from build123d import *

# Parameters (mm, degrees)
SKETCH1_W           = 944
SKETCH1_H           = 20
BOSS_EXTRUDE1_DEPTH = 204
CUT_EXTRUDE1_DEPTH  = 18
CUT_EXTRUDE2_DEPTH  = 2


with BuildPart() as part:
    # Sketch1 → Boss-Extrude1 (new body)
    with BuildSketch(Plane.XY):
        with Locations((393.099899989, 5.665003505)):
            Rectangle(SKETCH1_W, SKETCH1_H)
    extrude(amount=-BOSS_EXTRUDE1_DEPTH)

    # 3DSketch1 → Cut-Extrude1 (cut)
    with BuildSketch(Plane(origin=(863.099899989, 15.665003505, -202), x_dir=(-0.9781059289848355, 0, 0.2081076444648586), z_dir=(0, -1, 0))):
        Polygon((0, 0), (919.419573246, 195.621185797), (961.041102139, 0), (41.621528893, -195.621185797), align=None)
    extrude(amount=CUT_EXTRUDE1_DEPTH, mode=Mode.SUBTRACT)

    # 3DSketch2 → Cut-Extrude2 (cut)
    with BuildSketch(Plane(origin=(-58.900100011, -2.334996495, -184), x_dir=(0.9839394949368245, 0, 0.1785022977540257), z_dir=(0, -1, 0))):
        Polygon((0, 0), (889.481303423, -161.36607717), (918.755680255, 0), (29.274376832, 161.36607717), align=None)
    extrude(amount=CUT_EXTRUDE2_DEPTH, mode=Mode.SUBTRACT)


solid = part.part
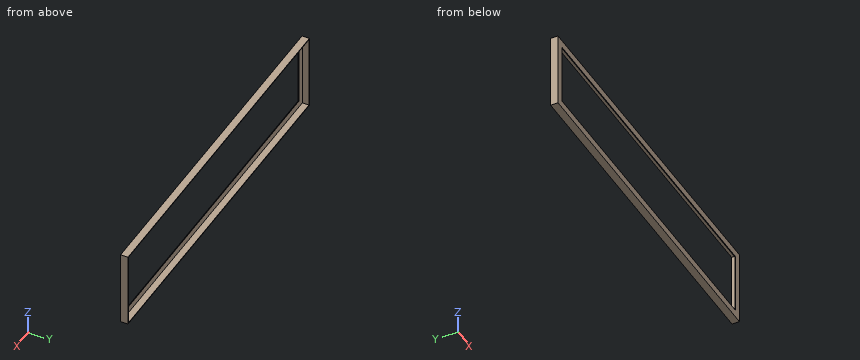
Could you check a few things on this model? Use its own coordinates, in mm. Give positions to 0.01 mm unless a question says otherwise; leave off trailing zeros. Write each loop counter-clockwise with the first axis right and the second up, starting at its lowest first coordinate (ties: lowest second). Pieces come first, ordered by that corner, then holes. Notation, with made-up numbers: (10, 8) -> (28, 8) arc R29 ccw to (28, 42) -> close; hole circle Ø3 at (-24.5, -25). An arc over 180 degrees is marked (long way). Write each question's results on one line, items separated by ' | '. Start each with the question number.
Q1. I need wall thicknesses on probe 1 along Z at (x, y) = (187.5, 12.5); probe 2 along X at (y, z) = (4, -84); probe 3 along X at (y, z) = (-2.75, -169). Which ranges of each line are inside material? Lowest first, please.
Q2. Suppose I cut it at B-B, the plane z = -97. List the corners of the cut face in (x, y) for me (3 decimals).
Q3. Suppose I cut it at A-A, the plane x = 599.5. List the corners of the cut face in (y, z) for me (3 decimals).
Q4. Suppose I cut it at C-C, the plane y = 11.5. List the corners of the cut face in (x, z) for me, and give its area (3 significant figures).
Outcome:
1) probe 1: -204 to -202, -2 to 0 | probe 2: -78.9 to -76.9, 863.1 to 865.1 | probe 3: -78.9 to -58.9, 845.1 to 865.1
2) outline: (-78.9, -4.335) -> (-58.9, -4.335) -> (-58.9, -2.335) -> (-76.9, -2.335) -> (-76.9, 15.665) -> (-78.9, 15.665) -> close; (845.1, -4.335) -> (865.1, -4.335) -> (865.1, 15.665) -> (863.1, 15.665) -> (863.1, -2.335) -> (845.1, -2.335) -> close
3) outline: (-4.335, -204) -> (15.665, -204) -> (15.665, -202) -> (-2.335, -202) -> (-2.335, -184) -> (-4.335, -184) -> close; (-4.335, -20) -> (-2.335, -20) -> (-2.335, -2) -> (15.665, -2) -> (15.665, 0) -> (-4.335, 0) -> close
4) outline: (-78.9, -204) -> (865.1, -204) -> (865.1, 0) -> (-78.9, 0) -> close; hole (-76.9, -202) -> (863.1, -202) -> (863.1, -2) -> (-76.9, -2) -> close | area: 4,580 mm2
